The drawing under review shows one solid part. Ordinate dimensions are in mm from its lowest x, y, z. Coordinates: 2 decimals unless noted, no trailing zeros. Loops run counter-clockwise (first coordinate to the right, second up) from the corner with the lowest first, then second, coordinate; pieces in that order, holes last. Notation, with made-up numbers: (32, -36) -> (90, -36) arc R29 ccw to (90, -16) -> close; hole circle Ø4 at (62, 3.25). An arc over 180 degrees is marked (long way). Use a Markdown table: item, result.
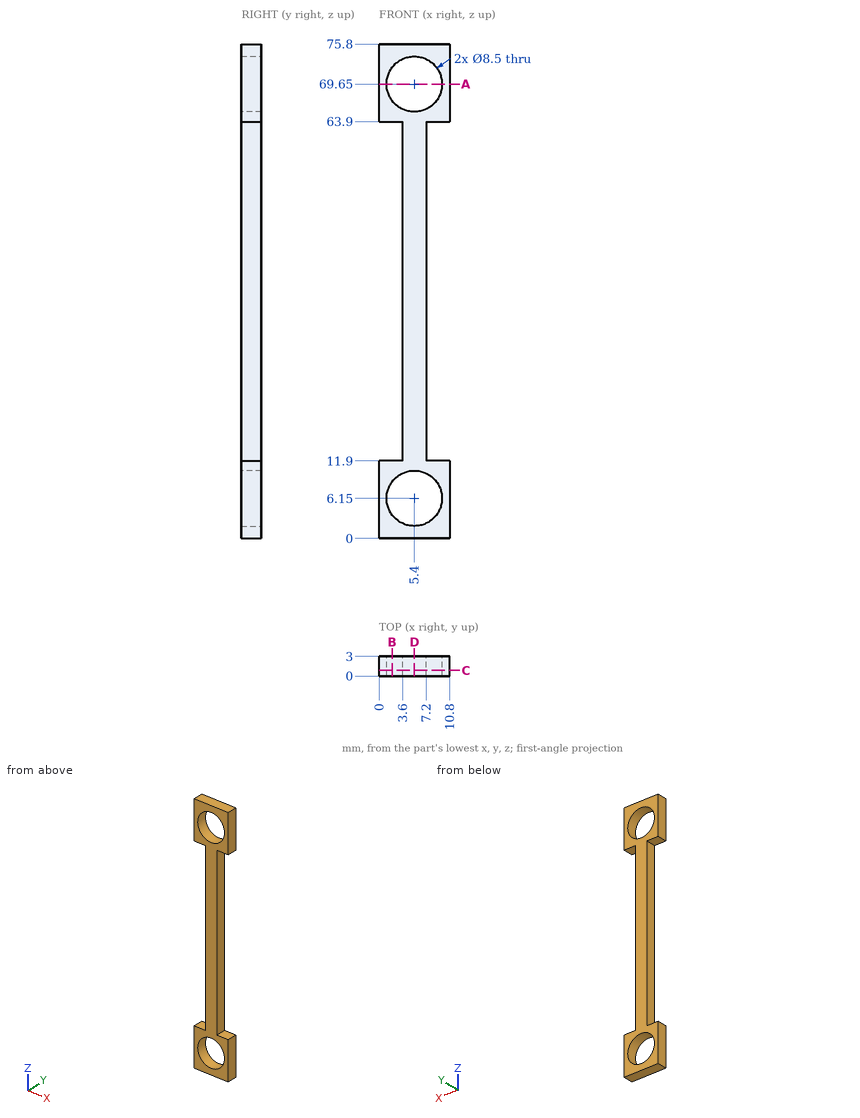
(1) For pin 1 Ø0.9 at (y, z) = (2, 46) entering from -X, flat-tipped, find the tip position at first contact; note if it passes through.
Found:
| item | result |
|---|---|
| pin 1 | stops at x = 3.6 |
(2) For line 1 along X through (y, z) = (1.6, 6.15); line 2 along Z through (x, y) = (6, 1.85); line 3 along Z through (x, y) = (10.25, 1.75), list the stretches that pass through material, from the lowest coordinate up.
Found:
| item | result |
|---|---|
| line 1 | x = 0 to 1.15, 9.65 to 10.8 |
| line 2 | z = 0 to 1.94, 10.36 to 65.44, 73.86 to 75.8 |
| line 3 | z = 0 to 11.9, 63.9 to 75.8 |
(3) Take a section at D-D on x = 5.4. Write out the cut boundary in (y, z).
Found:
| item | result |
|---|---|
| outline | (0, 0) -> (3, 0) -> (3, 1.9) -> (0, 1.9) -> close; (0, 10.4) -> (3, 10.4) -> (3, 65.4) -> (0, 65.4) -> close; (0, 73.9) -> (3, 73.9) -> (3, 75.8) -> (0, 75.8) -> close |
(4) Take a section at B-B on x = 2. Write out the cut boundary in (y, z), plus the area to 3 significant figures.
Found:
| item | result |
|---|---|
| outline | (0, 0) -> (3, 0) -> (3, 3.6) -> (0, 3.6) -> close; (0, 8.7) -> (3, 8.7) -> (3, 11.9) -> (0, 11.9) -> close; (0, 63.9) -> (3, 63.9) -> (3, 67.1) -> (0, 67.1) -> close; (0, 72.2) -> (3, 72.2) -> (3, 75.8) -> (0, 75.8) -> close |
| area | 40.8 mm^2 |
(5) Take a section at A-A on z = 69.65. Write out the cut boundary in (x, y).
Found:
| item | result |
|---|---|
| outline | (0, 0) -> (1.15, 0) -> (1.15, 3) -> (0, 3) -> close; (9.65, 0) -> (10.8, 0) -> (10.8, 3) -> (9.65, 3) -> close |
(6) Take a section at C-C on y = 0.85. Write out the cut boundary in (x, z).
Found:
| item | result |
|---|---|
| outline | (0, 0) -> (10.8, 0) -> (10.8, 11.9) -> (7.2, 11.9) -> (7.2, 63.9) -> (10.8, 63.9) -> (10.8, 75.8) -> (0, 75.8) -> (0, 63.9) -> (3.6, 63.9) -> (3.6, 11.9) -> (0, 11.9) -> close; hole circle Ø8.5 at (5.4, 6.15); hole circle Ø8.5 at (5.4, 69.65) |
